from build123d import *

# Parameters (mm, degrees)
SKETCH1_R           = 10
SKETCH1_W           = 10
SKETCH1_H           = 10
BOSS_EXTRUDE1_DEPTH = 5


with BuildPart() as part:
    # Sketch1 → Boss-Extrude1 (new body)
    with BuildSketch(Plane(origin=(0, 0, 0), x_dir=(1, 0, 0), z_dir=(0, 1, 0))):
        with BuildLine():
            Line((0, 0), (45, 0))
            Line((45, 0), (45, 25))
            Line((45, 25), (0, 25))
            ThreePointArc((0, 25), (-12.5, 12.5), (0, 0))
        make_face()
        with Locations(Location((0, 12.5, 0), (0, 0, 270))):
            Circle(SKETCH1_R, mode=Mode.SUBTRACT)
        with Locations((38, 12.5)):
            Rectangle(SKETCH1_W, SKETCH1_H, mode=Mode.SUBTRACT)
    extrude(amount=BOSS_EXTRUDE1_DEPTH)


solid = part.part
CAD build for the part. Positions are in the model's coordinates, mm. A direction names the side the tool comes from. Give positions to 0.01 mm unless a question says otherwise; leave off trailing zeros. Loops run counter-clockwise (first coordinate to the right, second up) from the corner with the lowest first, then second, coordinate; pieces in that order, holes last. Notation, with made-up numbers: M 81.5,31.5 L 118.5,31.5 A17 ccw 118.5,61.5 Z; hole C 24,38 d10. An arc over 180 degrees is marked long. Answer in a Markdown table with one row per item. Add a question column.
Item 1: Band-saw the part on D-D on z = -5.5. Give the cut face in (x, y), then the cut area to 3 significant figures.
Item 2: Tool access for faces 5 (the face through (22, 2, 0)), 6 (the face through (38, 2, -17.5)): list every direction of +Z, -Z, +X, -X, +Y, -Y with a clear straight run to the whole face (end or side of a thin tool).
Item 3: Band-saw the part on C-C on x = -5. Give the cut face in (y, z), then the cut area to 3 significant figures.
Item 4: Band-saw the part on A-A on y = 3.85. Give the cut face in (x, z).
Item 5: Mould opens along X. For faces 1 (the face through (38, 2, -7.5)), 2 (the face through (22, 5, -13)), 3 (the face through (43, 2, -12)), 4 (the face through (45, 2, -12)) say: +X half, -X half, draft (parallel to the pull), parting line (faces both ways), or undercut.
Item 6: Probe probe 1 along X at (y, z) = (3.85, -12.5); probe 2 along Z at (x, y) = (41.5, 3.15); probe 3 along X at (y, z) = (1.7, -9.25). List the from-to ranges inside material, lowest first.
Item 7: Band-saw the part on B-B on z = -12.5. Give the cut face in (x, y), then the cut area to 4 significant figures.
Item 8: Drop a flat-ended pin along its axis: P1, Ø1.5, axis at y = 3.5, z = -10.5, coming from the -X side. Give the stop position or say it passes through.
Reply:
| question | item | result |
|---|---|---|
| 1 | outline | M -10.36,0 L -7.14,0 L -7.14,5 L -10.36,5 Z; M 7.14,0 L 45,0 L 45,5 L 7.14,5 Z |
| 1 | area | 205 mm^2 |
| 2 | face 5 | +Z, +X, -X, +Y, -Y |
| 2 | face 6 | +Y, -Y |
| 3 | outline | M 0,-23.96 L 5,-23.96 L 5,-21.16 L 0,-21.16 Z; M 0,-3.84 L 5,-3.84 L 5,-1.04 L 0,-1.04 Z |
| 3 | area | 28.0 mm^2 |
| 4 | outline | M 0,-25 L 45,-25 L 45,0 L 0,0 A12.5 ccw Z; hole C 0,-12.5 d20; hole M 33,-17.5 L 43,-17.5 L 43,-7.5 L 33,-7.5 Z |
| 5 | face 1 | undercut |
| 5 | face 2 | draft |
| 5 | face 3 | undercut |
| 5 | face 4 | +X half |
| 6 | probe 1 | x = -12.5 to -10, 10 to 33, 43 to 45 |
| 6 | probe 2 | z = -25 to -17.5, -7.5 to 0 |
| 6 | probe 3 | x = -12.07 to -9.46, 9.46 to 33, 43 to 45 |
| 7 | outline | M -12.5,0 L -10,0 L -10,5 L -12.5,5 Z; M 10,0 L 33,0 L 33,5 L 10,5 Z; M 43,0 L 45,0 L 45,5 L 43,5 Z |
| 7 | area | 137.5 mm^2 |
| 8 | P1 | stops at x = -12.44 |
